Design review of the part built by this model. Coordinates are the model's own, in mm. A direction names the side the tool comes from. Coordinates: 2 decimals unless noted, no trailing zeros. Loops run counter-clockwise (first coordinate to the right, second up) from the corner with the lowest first, then second, coordinate; pieces in that order, holes last. Notation, with made-up numbers: (42, 0) -> (101, 0) arc R10 ccw to (101, 8) -> close; hole circle Ø3 at (-15, 20). An arc over 180 degrees is marked (long way). Use a Markdown table: item, result. Add a question column.
Q1. Take a section at A-A on z = -3.5. Write out the cut boundary in (x, y), plus the area to 3 significant figures.
Q2. Take a section at C-C on y = 6. Write out the cut boundary in (x, z).
Q3. Clearance check with flat-ended pins moving along their axes: pin 1 Ø2.5 at (x, y) = (22, -13) entering from +Z; pin 2 Ø0.8 at (x, z) = (23, -4) entering from -Y; pin 3 Ø5 at (x, y) = (17.5, -1.5) entering from +Z. State where each tip first meets the part, or that it passes through.
Q4. For faces 4 (the face through (25.25, 0, -4)), 5 (the face through (-18.5, 15, -5)), list the 3-axis set-ups (+Z, -Z, +X, -X, +Y, -Y) from which the entire face can be reached by the end or side of a thin tool; tool diameter is ignored.
Q5. For probe 1 along Y at (x, z) = (21.5, -4.7); probe 2 along X at (y, z) = (0, -0.75); probe 3 along Y at (x, z) = (1.5, -1.75), list the stretches that pass through material, from the lowest coordinate up.
Q6. Draft analysis for pull direction Y (two halves, no side actions). For faces 1 (the face through (0, 17, 0)), 2 (the face through (24.273, -16.323, -3.944)), 3 (the face through (19.36, 11.4, -4.88)), state which applies: pulls with the +Y half, pulls with the -Y half, needs draft (parallel to the pull), parting line crosses it, or undercut.
Q7. Take a section at B-B on x = 13. Write out the cut boundary in (y, z).
from build123d import *

# Parameters (mm, degrees)
PAD_DEPTH    = 8
THICKNESS_T  = -1.15
SKETCH002_R  = 1.6
PAD008_DEPTH = 4


with BuildPart() as part:
    # Sketch001 → Pad (new body)
    with BuildSketch(Plane.XY):
        with BuildLine():
            Line((-25.25, 14), (-25.25, -14))
            ThreePointArc((-25.25, -14), (-24.298097, -16.298097), (-22, -17.25))
            Line((-22, -17.25), (22, -17.25))
            ThreePointArc((22, -17.25), (24.298097, -16.298097), (25.25, -14))
            Line((25.25, -14), (25.25, 14))
            ThreePointArc((25.25, 14), (24.298097, 16.298097), (22, 17.25))
            Line((22, 17.25), (-22, 17.25))
            ThreePointArc((-22, 17.25), (-24.298097, 16.298097), (-25.25, 14))
        make_face()
    extrude(amount=-PAD_DEPTH)

    # Thickness
    thickness_openings = [part.faces().sort_by_distance(p)[0] for p in [
        (0, 0, 0),
    ]]
    offset(amount=THICKNESS_T, openings=thickness_openings)

    # Sketch002 (on Face19 of Thickness) → Pad008 (join)
    with BuildSketch(Plane.XY.offset(-6.85)):
        with BuildLine():
            Line((-24.1, 14), (-24.1, 10.5))
            Line((-24.1, 10.5), (-21.5, 10.5))
            ThreePointArc((-21.5, 10.5), (-19.37868, 11.37868), (-18.5, 13.5))
            Line((-18.5, 13.5), (-18.5, 16.1))
            Line((-18.5, 16.1), (-22, 16.1))
            ThreePointArc((-22, 16.1), (-23.484924, 15.484924), (-24.1, 14))
        make_face()
        with Locations((-21.5, 13.5)):
            Circle(SKETCH002_R, mode=Mode.SUBTRACT)
        with BuildLine():
            Line((18.5, 16.1), (18.5, 13.5))
            ThreePointArc((18.5, 13.5), (19.37868, 11.37868), (21.5, 10.5))
            Line((21.5, 10.5), (24.1, 10.5))
            Line((24.1, 10.5), (24.1, 14))
            ThreePointArc((24.1, 14), (23.484924, 15.484924), (22, 16.1))
            Line((22, 16.1), (18.5, 16.1))
        make_face()
        with Locations((21.5, 13.5)):
            Circle(SKETCH002_R, mode=Mode.SUBTRACT)
        with BuildLine():
            Line((-21.5, -10.5), (-24.1, -10.5))
            Line((-24.1, -10.5), (-24.1, -14))
            ThreePointArc((-24.1, -14), (-23.484924, -15.484924), (-22, -16.1))
            Line((-22, -16.1), (-18.5, -16.1))
            Line((-18.5, -16.1), (-18.5, -13.5))
            ThreePointArc((-18.5, -13.5), (-19.37868, -11.37868), (-21.5, -10.5))
        make_face()
        with Locations((-21.5, -13.5)):
            Circle(SKETCH002_R, mode=Mode.SUBTRACT)
        with BuildLine():
            Line((18.5, -13.5), (18.5, -16.1))
            Line((18.5, -16.1), (22, -16.1))
            ThreePointArc((22, -16.1), (23.484924, -15.484924), (24.1, -14))
            Line((24.1, -14), (24.1, -10.5))
            Line((24.1, -10.5), (21.5, -10.5))
            ThreePointArc((21.5, -10.5), (19.37868, -11.37868), (18.5, -13.5))
        make_face()
        with Locations((21.5, -13.5)):
            Circle(SKETCH002_R, mode=Mode.SUBTRACT)
    extrude(amount=PAD008_DEPTH)


solid = part.part
Answer list:
| question | item | result |
|---|---|---|
| 1 | outline | (-25.25, -14) arc R3.25 ccw to (-22, -17.25) -> (22, -17.25) arc R3.25 ccw to (25.25, -14) -> (25.25, 14) arc R3.25 ccw to (22, 17.25) -> (-22, 17.25) arc R3.25 ccw to (-25.25, 14) -> close; hole (-24.1, -10.5) -> (-21.5, -10.5) arc R3 cw to (-18.5, -13.5) -> (-18.5, -16.1) -> (18.5, -16.1) -> (18.5, -13.5) arc R3 cw to (21.5, -10.5) -> (24.1, -10.5) -> (24.1, 10.5) -> (21.5, 10.5) arc R3 cw to (18.5, 13.5) -> (18.5, 16.1) -> (-18.5, 16.1) -> (-18.5, 13.5) arc R3 cw to (-21.5, 10.5) -> (-24.1, 10.5) -> close; hole circle Ø3.2 at (-21.5, -13.5); hole circle Ø3.2 at (-21.5, 13.5); hole circle Ø3.2 at (21.5, -13.5); hole circle Ø3.2 at (21.5, 13.5) |
| 1 | area | 267 mm² |
| 2 | outline | (-25.25, -8) -> (25.25, -8) -> (25.25, 0) -> (24.1, 0) -> (24.1, -6.85) -> (-24.1, -6.85) -> (-24.1, 0) -> (-25.25, 0) -> close |
| 3 | pin 1 | z = -2.85 |
| 3 | pin 2 | y = -17.19 |
| 3 | pin 3 | z = -6.85 |
| 4 | face 4 | +Z, -Z, +X, +Y, -Y |
| 4 | face 5 | +Z |
| 5 | probe 1 | -17.25 to -15.1, -11.9 to -10.5, 10.5 to 11.9, 15.1 to 17.25 |
| 5 | probe 2 | -25.25 to -24.1, 24.1 to 25.25 |
| 5 | probe 3 | -17.25 to -16.1, 16.1 to 17.25 |
| 6 | face 1 | needs draft |
| 6 | face 2 | pulls with the -Y half |
| 6 | face 3 | undercut |
| 7 | outline | (-17.25, -8) -> (17.25, -8) -> (17.25, 0) -> (16.1, 0) -> (16.1, -6.85) -> (-16.1, -6.85) -> (-16.1, 0) -> (-17.25, 0) -> close |
